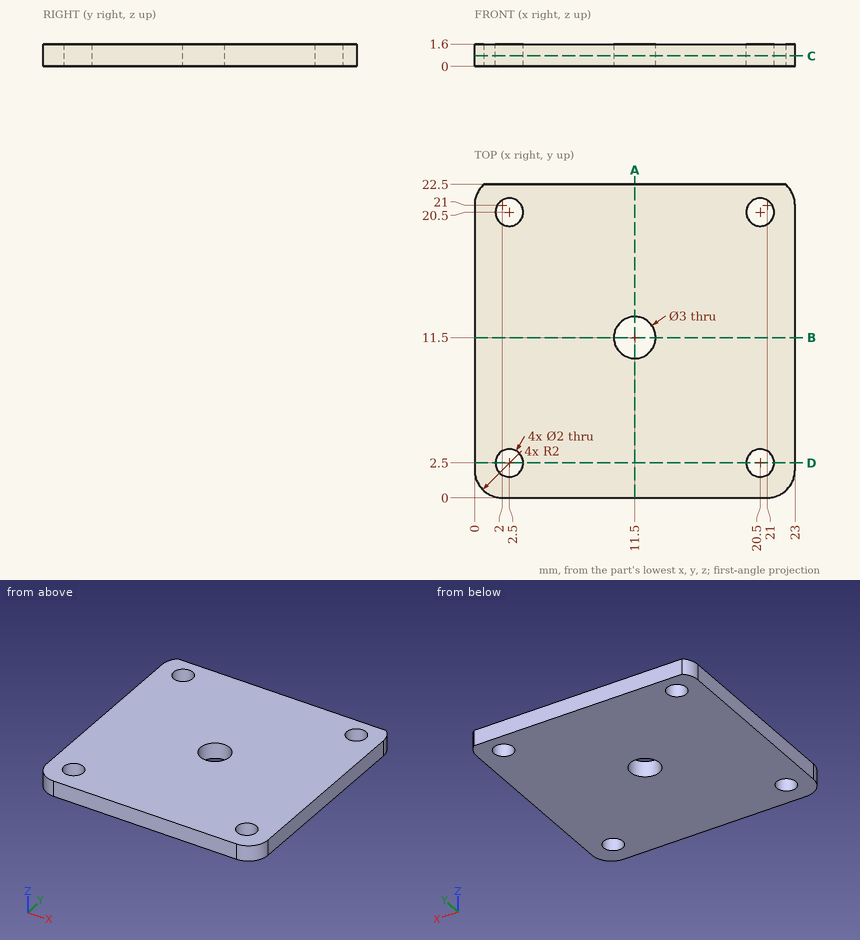
The figure shows three views and two pictorial views of one solid part (mm, origin at its lowest corner). Answer the questions. Coordinates: 2 decimals unless noted, no trailing zeros. Write each loop counter-clockwise with the first axis right and the second up, starting at its lowest first coordinate (ties: lowest second). Pieces come first, ordered by that corner, then holes. Notation, with made-up numbers: (-5, 50) -> (17, 50) arc R22 ccw to (17, 65) -> close; hole circle Ø4 at (-32, 2.25). An arc over 180 degrees is marked (long way). Return JSON: item names as keys, results as strings.
1. A cutting plane is placed at A-A (x = 11.5). Determine the outline of the cut face in (y, z), and give its area (3 significant figures).
Found:
{"outline": "(0, 0) -> (10, 0) -> (10, 1.6) -> (0, 1.6) -> close; (13, 0) -> (22.5, 0) -> (22.5, 1.6) -> (13, 1.6) -> close", "area": "31.2 mm2"}
2. Find the intervals of material crossed by line 1 along Y through (x, z) = (2.5, 1.15); line 2 along Y through (x, z) = (20, 1.05); line 3 along Y through (x, z) = (11.5, 0.75), in increasing order. Write a range as from..to.
Found:
{"line 1": "0..1.5, 3.5..19.5, 21.5..22.5", "line 2": "0..1.63, 3.37..19.63, 21.37..22.5", "line 3": "0..10, 13..22.5"}
3. A cutting plane is placed at C-C (z = 0.75). Determine the outline of the cut face in (x, y), and give its area (3 significant figures).
Found:
{"outline": "(0, 2) arc R2 ccw to (2, 0) -> (21, 0) arc R2 ccw to (23, 2) -> (23, 21) arc R2 ccw to (22.32, 22.5) -> (0.68, 22.5) arc R2 ccw to (0, 21) -> close; hole circle Ø2 at (2.5, 2.5); hole circle Ø2 at (2.5, 20.5); hole circle Ø3 at (11.5, 11.5); hole circle Ø2 at (20.5, 2.5); hole circle Ø2 at (20.5, 20.5)", "area": "496 mm2"}
4. A cutting plane is placed at D-D (y = 2.5). Determine the outline of the cut face in (x, z), and give its area (3 significant figures).
Found:
{"outline": "(0, 0) -> (1.5, 0) -> (1.5, 1.6) -> (0, 1.6) -> close; (3.5, 0) -> (19.5, 0) -> (19.5, 1.6) -> (3.5, 1.6) -> close; (21.5, 0) -> (23, 0) -> (23, 1.6) -> (21.5, 1.6) -> close", "area": "30.4 mm2"}
5. A cutting plane is placed at B-B (y = 11.5). Determine the outline of the cut face in (x, z), and give its area (3 significant figures).
Found:
{"outline": "(0, 0) -> (10, 0) -> (10, 1.6) -> (0, 1.6) -> close; (13, 0) -> (23, 0) -> (23, 1.6) -> (13, 1.6) -> close", "area": "32.0 mm2"}
6. This flat-tipped pin is pushed along its axis until it touches: P1, Ø4, axis at x = 11.5, y = 11.5, coming from the +Z side. Where does it stop, or does it pass through?
Found:
{"P1": "z = 1.6"}
